Job drawing, mm, ordinate dimensions from the low corner. One solid piece. A direction names the side the tool comes from. Coordinates: 2 decimals unless noted, no trailing zeros. Order: outer loops, then holes, each group sorted by start corner. A loop starts at its lowest first (then second) coordinate and runs counter-clockwise, first axis right, second up. Notation, with made-up numbers: (79, 58.5) -> (98, 58.5) arc R12 cw to (98, 68.5) -> close; hole circle Ø5 at (18, -15.5). An arc over 180 degrees is marked (long way). Use CSV: the item, a comma, the result in double quotes. Start each with the question number.
(1) Cut at A-A on z = 12.7. Write the cut outline in (x, y) (1 decimal), plus the area to 3 significant figures.
(2) Probe L1, parallel to X at y = 19.75, z = 12.7; L2, parallel to Y at x = 22.75, z = 15.5. List the from-to ranges inside material, lowest first.
(3) Tool access for the marked faces 1 and 2: list every direction of +Z, -Z, +X, -X, +Y, -Y with a clear straight run to the whole face (end or side of a thin tool).
(4) Cut at C-C on y = 11.25. Write the cut outline in (x, z), plus the area to 3 significant figures.
(5) Pin check, flat tips, straight feed: pin 1 Ø1 at (x, y) = (6, 7) entering from -Z; pin 2 Ø10 at (x, y) = (22, 11.5) entering from -Z; pin 3 Ø1.5 at (x, z) = (12, 3.5) entering from +Y. Stop position of each tip, or through.
(6) Cut at B-B on x = 12.7. Write the cut outline in (y, z) (1 decimal), plus the area to 3 significant figures.
(7) Cut at D-D on z = 7. Write the cut outline in (x, y) (1 decimal).
(8) Pull direction X, two halves, no side cores. Call the marked faces 3, 4 and 5: pulls with the +X half, pulls with the -X half, needs draft (parallel to the pull), parting line crosses it, or undercut.
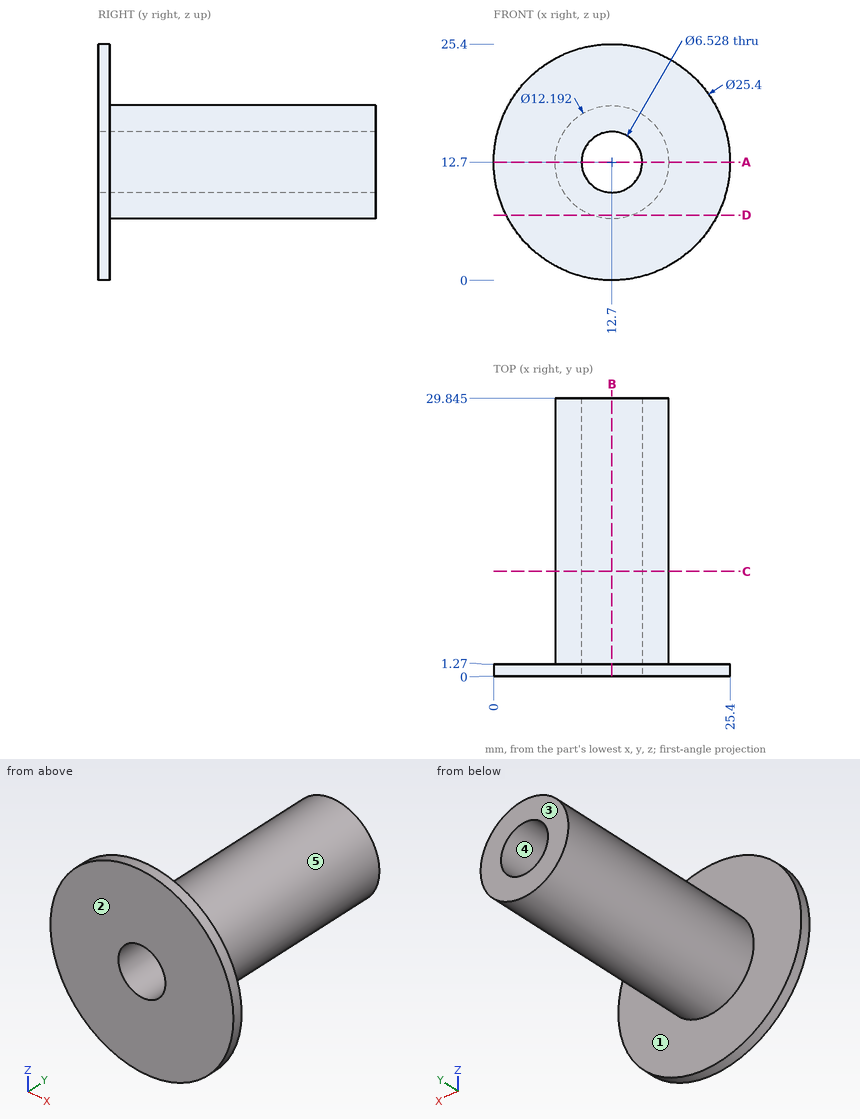
Outcome:
1,outline,"(0, 0) -> (9.4, 0) -> (9.4, 29.8) -> (6.6, 29.8) -> (6.6, 1.3) -> (0, 1.3) -> close; (16, 0) -> (25.4, 0) -> (25.4, 1.3) -> (18.8, 1.3) -> (18.8, 29.8) -> (16, 29.8) -> close"
1,area,"186 mm2"
2,L1,"6.6 to 9.44, 15.96 to 18.8"
2,L2,"0 to 1.27"
3,face 1,"+Y"
3,face 2,"+Z, -Z, +X, -X, -Y"
4,outline,"circle Ø12.19 at (12.7, 12.7); hole circle Ø6.53 at (12.7, 12.7)"
4,area,"83.3 mm2"
5,pin 1,"through"
5,pin 2,"z = 8.38"
5,pin 3,"y = 1.27"
6,outline,"(0, 0) -> (1.3, 0) -> (1.3, 6.6) -> (29.8, 6.6) -> (29.8, 9.4) -> (0, 9.4) -> close; (0, 16) -> (29.8, 16) -> (29.8, 18.8) -> (1.3, 18.8) -> (1.3, 25.4) -> (0, 25.4) -> close"
6,area,"186 mm2"
7,outline,"(1.4, 0) -> (24, 0) -> (24, 1.3) -> (14.9, 1.3) -> (14.9, 29.8) -> (10.5, 29.8) -> (10.5, 1.3) -> (1.4, 1.3) -> close"
8,face 3,"needs draft"
8,face 4,"undercut"
8,face 5,"parting line crosses it"
